Geometry check sheet. Reference: drawing and pictorial views, mm from the part's lowest x, y, z. A direction names the side the tool comes from. Round coordinates to 2 decimals unless told otherwise and drop trailing zeros. Write each loop counter-clockwise with the first axis right and the second up, starting at its lowest first coordinate (ties: lowest second). Pieces come first, ordered by that corner, then holes. Notation, with made-up numbers: (12.5, 19.25) - (37.5, 19.25) arc R17 ccw to (37.5, 35.25) - close; hole circle Ø1 at (-1.75, 58.25). An arc over 180 degrees is marked (long way). Return JSON: item names as keys, results as strings.
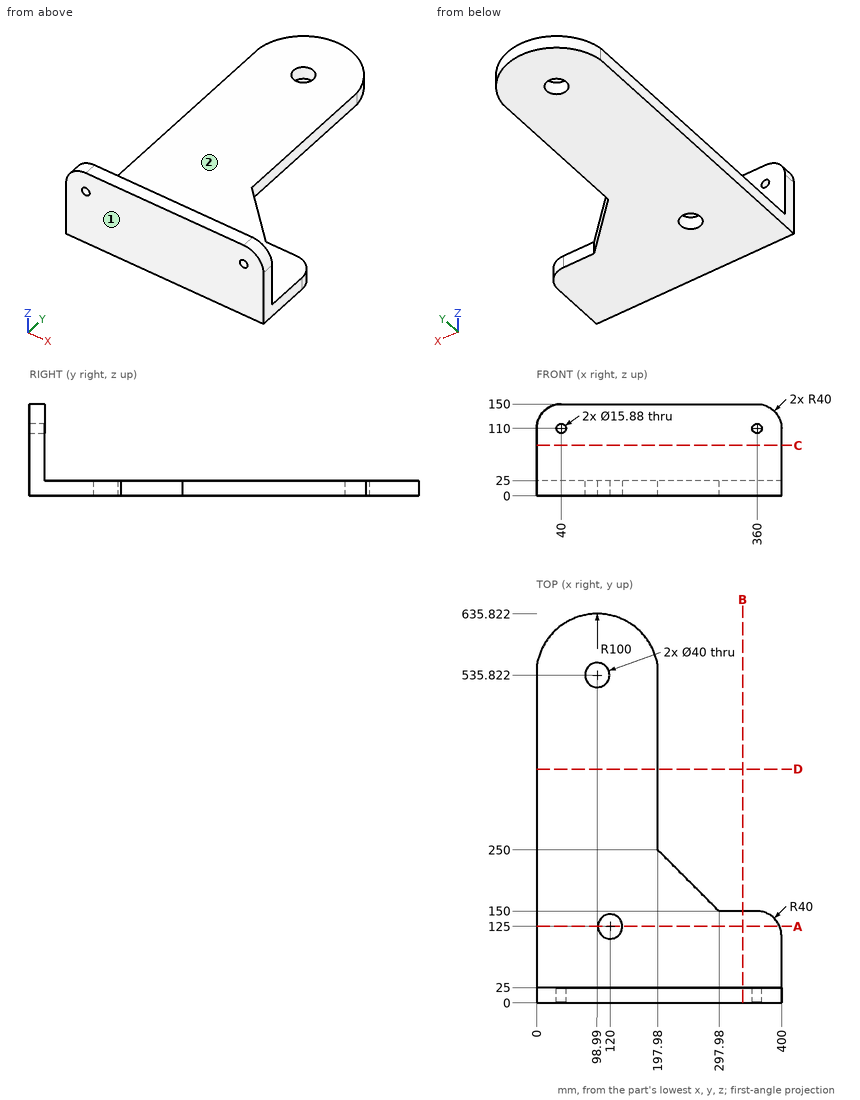
(1) Section check A-A, the plane y = 125. Enter the section's corners in (x, z).
Response values:
{"outline": "(0, 0) - (100, 0) - (100, 25) - (0, 25) - close; (140, 0) - (397.08, 0) - (397.08, 25) - (140, 25) - close"}
(2) Material ranges on line 1 along X through (y, z) = (10.5, 110); line 2 along Z through (x, y) = (360, 6.25); line 3 along Z through (x, y) = (47.5, 376), recorded low to high. Write a range as [from, to].
Response values:
{"line 1": "x = [0, 32.06], [47.94, 352.06], [367.94, 400]", "line 2": "z = [0, 102.06], [117.94, 150]", "line 3": "z = [0, 25]"}
(3) Gauge pin test, flat ends, axial feed: pin 1 (12 mm diameter, centred on y = 239.5, z = 16.5, fed in from +X); pin 2 (7.5 mm diameter, centred on x = 340, z = 7, fed in from +Y); pin 3 (4 mm diameter, centred on x = 155.5, y = 307.5, fed in from +Z); pin 4 (18.5 mm diameter, centred on x = 40, z = 110, fed in from -Y). Record the tip position at first contact, or that the pin passes through.
Response values:
{"pin 1": "stops at x = 214.48", "pin 2": "stops at y = 150", "pin 3": "stops at z = 25", "pin 4": "stops at y = 0"}
(4) Section check B-B, the plane x = 336.5. Enter the section's corners in (y, z).
Response values:
{"outline": "(0, 0) - (150, 0) - (150, 25) - (25, 25) - (25, 150) - (0, 150) - close"}
(5) Section check D-D, the plane y = 382. Enter the section's corners in (x, z), plus the area to 3 significant figures.
Response values:
{"outline": "(0, 0) - (197.98, 0) - (197.98, 25) - (0, 25) - close", "area": "4,950 mm^2"}
(6) Access from +Z, -Z, +X, -X, +Y, -Y to the whole of each face (thin tool, end or side, straight path). Record for the marked faces 1 and 2.
Response values:
{"face 1": "+Z, -Z, +X, -X, -Y", "face 2": "+Z, +X, -X, +Y"}
(7) Section check C-C, the plane z = 82.5. Enter the section's corners in (x, y), plus the area to 4 significant figures.
Response values:
{"outline": "(0, 0) - (400, 0) - (400, 25) - (0, 25) - close", "area": "10,000 mm^2"}
